The figure shows three views and two pictorial views of one solid part (mm, origin at its lowest corner). Answer the questions. A direction names the side the tool comes from. Give positions to 0.01 mm unless a question says otherwise; leave off trailing zeros. Write each loop counter-clockwise with the first axis right and the second up, starting at its lowest first coordinate (ties: lowest second). Pieces come first, ordered by that corner, then holes. Notation, with made-up numbers: (22, -6) - (72, -6) arc R26 ccw to (72, 15) - close; hole circle Ø6 at (-37, -0.75). An arc over 180 degrees is marked (long way). Use a Markdown table: item, result. Add a question column.
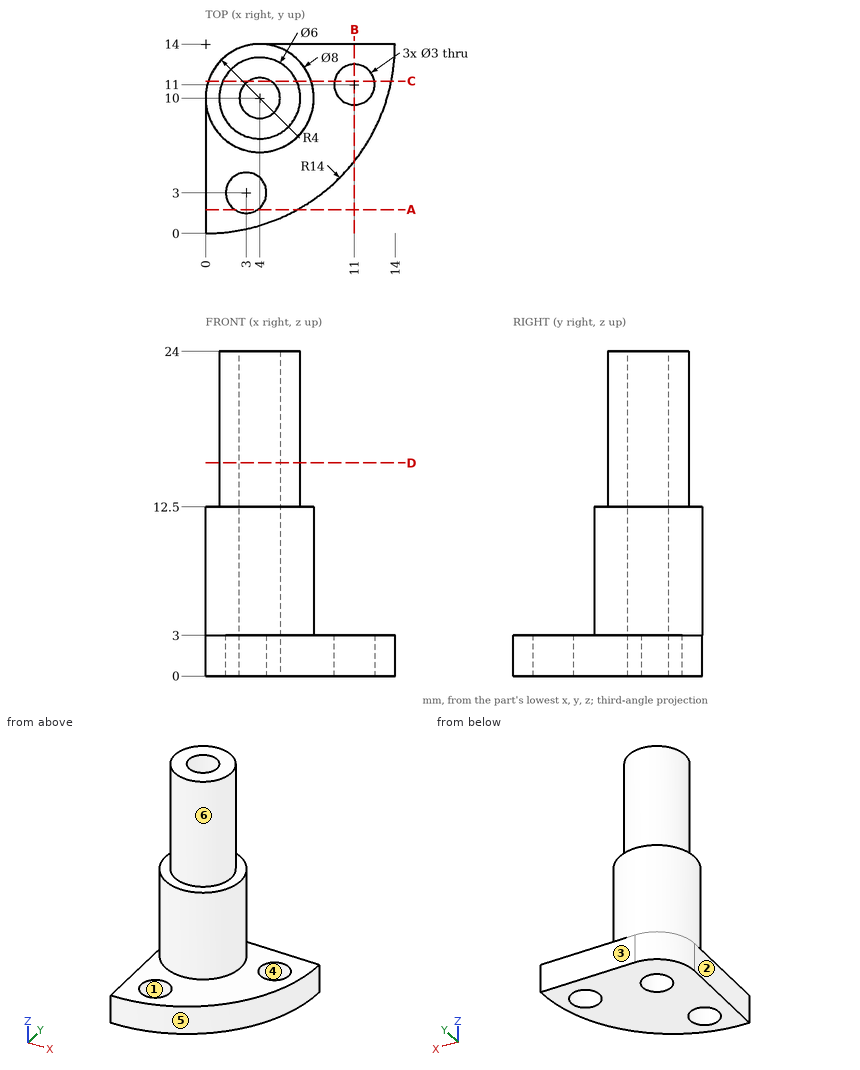
1. The part is cut by section D-D (z = 15.75). Give the vertices of the cut face in (x, y), and give its area (3 significant figures).
2. Which of the six approach directions +Z, -Z, +X, -X, +Y, -Y give full straight-line access (tool end or side, diameter ignored) to the marked faces 5 and 6?
3. The part is cut by section B-B (x = 11). Give the vertices of the cut face in (y, z), and give its area (3 significant figures).
4. Given P1, Ø3, axis at y = 6, z = 15, coming from the -X side; P2, Ø4, axis at y = 8.5, z = 8, coming from the +X side; P3, Ø2, axis at x = 1.5, z = 19, coming from the +Y side, each flat-ended and moving along its own axis, determine where each tip first touches the part or whether it passes through.
5. The part is cut by section A-A (y = 1.75). Give the vertices of the cut face in (x, z), and give its area (3 significant figures).
6. Consider L1, parallel to Y at x = 3, z = 1.15; L2, parallel to Y at x = 4, z = 14.5; L3, parallel to Y at x = 4, z = 7.75. Determine where each line is inside the solid, lowest interval first. Write a range as [from, to].
7. The part is cut by section C-C (y = 11.25). Give the vertices of the cut face in (x, z), and give its area (3 significant figures).
8. For a pull along Y with two mould halves and no side action, classify the marked faces 1, 2, 3 and 4 as released by +Y, released by -Y, zero draft, split by the parting line, or undercut.
Check values:
| question | item | result |
|---|---|---|
| 1 | outline | circle Ø6 at (4, 10); hole circle Ø3 at (4, 10) |
| 1 | area | 21.2 mm2 |
| 2 | face 5 | +Z, -Z, +X, -Y |
| 2 | face 6 | +Z |
| 3 | outline | (5.34, 0) - (9.5, 0) - (9.5, 3) - (5.34, 3) - close; (12.5, 0) - (14, 0) - (14, 3) - (12.5, 3) - close |
| 3 | area | 17.0 mm2 |
| 4 | P1 | stops at x = 2.34 |
| 4 | P2 | stops at x = 8 |
| 4 | P3 | stops at y = 12.6 |
| 5 | outline | (0, 0) - (2.17, 0) - (2.17, 3) - (0, 3) - close; (3.83, 0) - (6.78, 0) - (6.78, 3) - (3.83, 3) - close |
| 5 | area | 15.4 mm2 |
| 6 | L1 | y = [0.33, 1.5], [4.5, 8.88], [11.12, 13.87] |
| 6 | L2 | y = [7, 8.5], [11.5, 13] |
| 6 | L3 | y = [6, 8.5], [11.5, 14] |
| 7 | outline | (0.2, 0) - (3.17, 0) - (3.17, 24) - (1.27, 24) - (1.27, 12.5) - (0.2, 12.5) - close; (4.83, 0) - (9.52, 0) - (9.52, 3) - (7.8, 3) - (7.8, 12.5) - (6.73, 12.5) - (6.73, 24) - (4.83, 24) - close; (12.48, 0) - (13.73, 0) - (13.73, 3) - (12.48, 3) - close |
| 7 | area | 127 mm2 |
| 8 | face 1 | undercut |
| 8 | face 2 | zero draft |
| 8 | face 3 | released by +Y |
| 8 | face 4 | undercut |
